Build history of the part. All positions in model axes, mm. A direction names the side the tool comes from. Coordinates: 2 decimals unless noted, no trailing zeros. Write each loop counter-clockwise with the first axis right and the second up, starting at its lowest first coordinate (ties: lowest second). Pieces come first, ordered by that corner, then holes.
from build123d import *

# Parameters (mm, degrees)
BOSS_EXTRU_1_DEPTH      = 100
ENL_V_MAT_EXTRU_1_DEPTH = 36


with BuildPart() as part:
    # Esquisse1 → Boss.-Extru.1 (new body)
    with BuildSketch(Plane.XY):
        with BuildLine():
            Line((-9, -15), (9, -15))
            ThreePointArc((9, -15), (11.121320344, -14.121320344), (12, -12))
            Line((12, -12), (12, 12))
            ThreePointArc((12, 12), (11.121320344, 14.121320344), (9, 15))
            Line((9, 15), (-9, 15))
            ThreePointArc((-9, 15), (-11.121320344, 14.121320344), (-12, 12))
            Line((-12, 12), (-12, -12))
            ThreePointArc((-12, -12), (-11.121320344, -14.121320344), (-9, -15))
        make_face()
        with BuildLine():
            Line((-7, -13), (7, -13))
            ThreePointArc((7, -13), (9.121320344, -12.121320344), (10, -10))
            Line((10, -10), (10, 10))
            ThreePointArc((10, 10), (9.121320344, 12.121320344), (7, 13))
            Line((7, 13), (-7, 13))
            ThreePointArc((-7, 13), (-9.121320344, 12.121320344), (-10, 10))
            Line((-10, 10), (-10, -10))
            ThreePointArc((-10, -10), (-9.121320344, -12.121320344), (-7, -13))
        make_face(mode=Mode.SUBTRACT)
    extrude(amount=-BOSS_EXTRU_1_DEPTH)

    # Esquisse2 → Enlèv. mat.-Extru.1 (cut)
    with BuildSketch(Plane(origin=(12, 0, 0), x_dir=(0, 0, -1), z_dir=(1, 0, 0))):
        with BuildLine():
            Line((92, -5.25), (8, -5.25))
            ThreePointArc((8, -5.25), (2.75, 0), (8, 5.25))
            Line((8, 5.25), (92, 5.25))
            ThreePointArc((92, 5.25), (97.25, 0), (92, -5.25))
        make_face()
    extrude(amount=-ENL_V_MAT_EXTRU_1_DEPTH, mode=Mode.SUBTRACT)


solid = part.part
(1) Slice it at B-B, the plane x = -3.25. List the corners of the cut face in (y, z).
(2) Slice it at A-A, the plane y = 0. List the corners of the cut face in (x, z).
(3) Slice it at D-D, the plane y = 7. List the corners of the cut face in (x, z).
(4) 3-axis set-ups, long thin cutter, end or side, ignore diameter. For faces 1 (the cylindrical face through (-9.1, 12.14, -49.3)), 2 (the flat face through (10.5, 0.2, 0)), 3 (the flat face through (-11, -5.25, -51)): which of +Z, -Z, +X, -X, +Y, -Y reach the whole face in a straight line?
(5) Slice it at C-C, the plane z = -64. List the corners of the cut face in (x, y).
(6) Probe L1, parallel to X at y = -8.25, z = -29.5; L2, parallel to Y at x = -3.5, z = -20.5; L3, parallel to X at y = -12.5, z = -60. List the from-to ranges inside material, lowest first.
(7) Flat gauge pins, fed straight in: P1, Ø1.6, axis at x = -11, z = -56, coming from the +Y side; P2, Ø1.6, axis at x = 11, z = -51.5, coming from the -Y side; P3, Ø2, axis at x = -11.5, z = -41.5, coming from the -Y side; P4, Ø6, axis at x = 6, y = -1, coming from the -Z side. Where does each tip first touch, or does it go through?
(8) Two-plate mould, pull along Y, no slides. Class faces 4 (the cylindrical face through (11.1, -14.14, -49.3)), 5 (the flat face through (0, 15, -49)), 6 (the flat face through (11, -5.25, -51)), 7 (the flat face through (12, -6, -49)): pulls with the +Y half, pulls with the -Y half, needs draft (parallel to the pull), parting line crosses it, or undercut.
Results:
1. outline: (-15, -100) - (-13, -100) - (-13, 0) - (-15, 0) - close; (13, -100) - (15, -100) - (15, 0) - (13, 0) - close
2. outline: (-12, -100) - (-10, -100) - (-10, -97.25) - (-12, -97.25) - close; (-12, -2.75) - (-10, -2.75) - (-10, 0) - (-12, 0) - close; (10, -100) - (12, -100) - (12, -97.25) - (10, -97.25) - close; (10, -2.75) - (12, -2.75) - (12, 0) - (10, 0) - close
3. outline: (-12, -100) - (-10, -100) - (-10, 0) - (-12, 0) - close; (10, -100) - (12, -100) - (12, 0) - (10, 0) - close
4. face 1: +Z, -Z
4. face 2: +Z, +X, -X, +Y, -Y
4. face 3: +X, -X
5. outline: (-12, -12) arc R3 ccw to (-9, -15) - (9, -15) arc R3 ccw to (12, -12) - (12, -5.25) - (10, -5.25) - (10, -10) arc R3 cw to (7, -13) - (-7, -13) arc R3 cw to (-10, -10) - (-10, -5.25) - (-12, -5.25) - close; (-12, 5.25) - (-10, 5.25) - (-10, 10) arc R3 cw to (-7, 13) - (7, 13) arc R3 cw to (10, 10) - (10, 5.25) - (12, 5.25) - (12, 12) arc R3 ccw to (9, 15) - (-9, 15) arc R3 ccw to (-12, 12) - close
6. L1: x = -12 to -10, 10 to 12
6. L2: y = -15 to -13, 13 to 15
6. L3: x = -11.96 to -8.66, 8.66 to 11.96
7. P1: stops at y = 14.75
7. P2: stops at y = -14.75
7. P3: stops at y = -14.6
7. P4: passes through
8. face 4: pulls with the -Y half
8. face 5: pulls with the +Y half
8. face 6: undercut
8. face 7: needs draft
